```python
from build123d import *

# Parameters (mm, degrees)
F1_DEPTH = 10
F2_DEPTH = 30
F3_R     = 0.99999


# Not quite as in the source:
# - a fillet or chamfer is up to 0.001 mm smaller than in the source, because OpenCascade refuses the exact size


with BuildPart() as f1:
    # F0 (on Top) → F1 (new body)
    with BuildSketch(Plane.XY):
        with BuildLine():
            ThreePointArc((-9.4454545455, 2.9653648055), (-9.7857038582, 1.5), (-9.9, 0))
            ThreePointArc((-9.9, 0), (-9.896558825, -0.0741336209), (-9.895411401, -0.1483381952))
            ThreePointArc((-9.895411401, -0.1483381952), (-9.8958382083, -0.193598479), (-9.8971184787, -0.238842665))
            ThreePointArc((-9.8971184787, -0.238842665), (-9.7668963107, -1.6179420433), (-9.4454545455, -2.9653648055))
            ThreePointArc((-9.4454545455, -2.9653648055), (0.0988831148, -9.8995061558), (9.5028042321, -2.7760964907))
            Line((9.5028042321, -2.7760964907), (7.3082145562, -3))
            ThreePointArc((7.3082145562, -3), (-7.9, 0), (7.3082145562, 3))
            Line((7.3082145562, 3), (9.3680287257, 3.2015680213))
            ThreePointArc((9.3680287257, 3.2015680213), (-0.1242846699, 9.8992198339), (-9.4454545455, 2.9653648055))
        make_face()
        with BuildLine():
            ThreePointArc((-9.4454545455, 2.9653648055), (-10.6009515165, 2.3129966374), (-11.9248231248, 2.2228775962))
            ThreePointArc((-11.9248231248, 2.2228775962), (-10.5211552877, 1.4678348291), (-9.9, 0))
            ThreePointArc((-9.9, 0), (-9.7857038582, 1.5), (-9.4454545455, 2.9653648055))
        make_face()
        with BuildLine():
            ThreePointArc((-9.8971184787, -0.238842665), (-10.4571434039, -1.6913128454), (-11.7905485927, -2.4946360333))
            ThreePointArc((-11.7905485927, -2.4946360333), (-10.5690595937, -2.4861794722), (-9.4454545455, -2.9653648055))
            ThreePointArc((-9.4454545455, -2.9653648055), (-9.7668963107, -1.6179420433), (-9.8971184787, -0.238842665))
        make_face()
    extrude(amount=F1_DEPTH)

    # F0 (on Top) → F2 (join)
    with BuildSketch(Plane.XY):
        with BuildLine():
            ThreePointArc((-9.9, 0), (-10.5211552877, 1.4678348291), (-11.9248231248, 2.2228775962))
            ThreePointArc((-11.9248231248, 2.2228775962), (-14.6944398213, -0.2166217115), (-11.7905485927, -2.4946360333))
            ThreePointArc((-11.7905485927, -2.4946360333), (-10.4571434039, -1.6913128454), (-9.8971184787, -0.238842665))
            ThreePointArc((-9.8971184787, -0.238842665), (-9.8992795935, -0.1194300232), (-9.9, 0))
        make_face()
    extrude(amount=F2_DEPTH)

    # F3 (radius 1 in the source; OpenCascade refuses exactly that, so slightly less here)
    f3_edges = [f1.edges().sort_by_distance(p)[0] for p in [
        (9.502804, -2.776096, 5),
        (7.308215, -3, 5),
        (9.368029, 3.201568, 5),
        (7.308215, 3, 5),
    ]]
    fillet(f3_edges, radius=F3_R)


solid = f1.part
```
Work out the finished part from the listing and answer in its coordinate system (mm). A direction names the side the tool comes from. Give positions to 0.01 mm unless a question says otherwise; leave off trailing zeros. Order: outer loops, then holes, each group sorted by start corner. A loop starts at its lowest first (then second) coordinate and runs counter-clockwise, first axis right, second up. Notation, with made-up numbers: (60, -19.75) - (94, -19.75) arc R5 ccw to (94, -12.75) - close; hole circle Ø8 at (78.5, -35). An arc over 180 degrees is marked (long way). One line per item, written item: value. Start each with the question number.
1. Each of these flat-tipped pins is pushed along its axis until it touches: pin 1 Ø6 at (x, y) = (-4, 5) entering from +Z; pin 2 Ø6 at (x, z) = (-11.5, 26.5) entering from -Y; pin 3 Ø6 at (y, z) = (-6, 5.5) entering from +X; pin 4 Ø8 at (y, z) = (-3.5, 24.5) entering from +X. Where does it stop, or does it pass through?
2. Which of the six approach directions +Z, -Z, +X, -X, +Y, -Y give full straight-line access (tool end or side, diameter ignored) to faces 4 (the face through (7.43, 3.19, 5.07)), 5 (the face through (-0.677, 9.877, 4.93))?
3. Consider line 1 (Y direction, x = 0, z = 5.5); line 2 (X direction, y = 6.75, z = 2); line 3 (Z direction, x = -7.25, y = -5.5). Determine where each line is inside the solid, lowest interval first.
4. Section B-B, the plane y = -7.25 is taken. Write down the section's boundary in (x, z), then the cut area to 3 significant figures.
5. Section D-D, the plane z = 13.75 is taken. Write down the section's boundary in (x, y), then the cut area to 3 significant figures.
6. Section A-A, the plane x = 0 is taken. Write down the section's boundary in (y, z).
7. For a pull along Y with two mould halves and no side action, classify faces 1 (the face through (-7.89, -0.36, 4.93)), 2 (the face through (-10.586, -2.483, 4.93)), 3 (the face through (-12, 0, 30)) as released by +Y, released by -Y, zero draft, split by the parting line, or undercut.
8. Section C-C, the plane y = -1 is taken. Write down the section's boundary in (x, z).
Filled sheet:
1. pin 1: z = 10
1. pin 2: y = -2.55
1. pin 3: x = 8.98
1. pin 4: x = -9.9
2. face 4: +Z, -Z
2. face 5: +Z, -Z, +Y
3. line 1: -9.9 to -7.9, 7.9 to 9.9
3. line 2: -7.24 to -4.1, 4.1 to 7.24
3. line 3: 0 to 10
4. outline: (-6.74, 0) - (-3.14, 0) - (-3.14, 10) - (-6.74, 10) - close; (3.14, 0) - (6.74, 0) - (6.74, 10) - (3.14, 10) - close
4. area: 72.1 mm²
5. outline: (-9.9, -0.24) arc R9.9 cw to (-9.9, 0) arc R2.4 ccw (long way) to start
5. area: 18.1 mm²
6. outline: (-9.9, 0) - (-7.9, 0) - (-7.9, 10) - (-9.9, 10) - close; (7.9, 0) - (9.9, 0) - (9.9, 10) - (7.9, 10) - close
7. face 1: undercut
7. face 2: released by -Y
7. face 3: zero draft
8. outline: (-14.54, 0) - (-7.84, 0) - (-7.84, 10) - (-10.05, 10) - (-10.05, 30) - (-14.54, 30) - close
